Part print with two shaded views. Sizes in mm from the minimum x, y, z corner. A direction names the side the tool comes from. Give positions to 0.01 mm unless a question says otherwise; leave off trailing zeros. Loops run counter-clockwise (first coordinate to the right, second up) from the corner with the lowest first, then second, coordinate; pieces in that order, holes last. Notation, with made-up numbers: (-34, 26.5) -> (-25, 26.5) arc R22 cw to (-25, 38.5) -> close; hole circle Ø2 at (10, 87). An arc over 180 degrees is marked (long way). One line per question, with ' | ' between items.
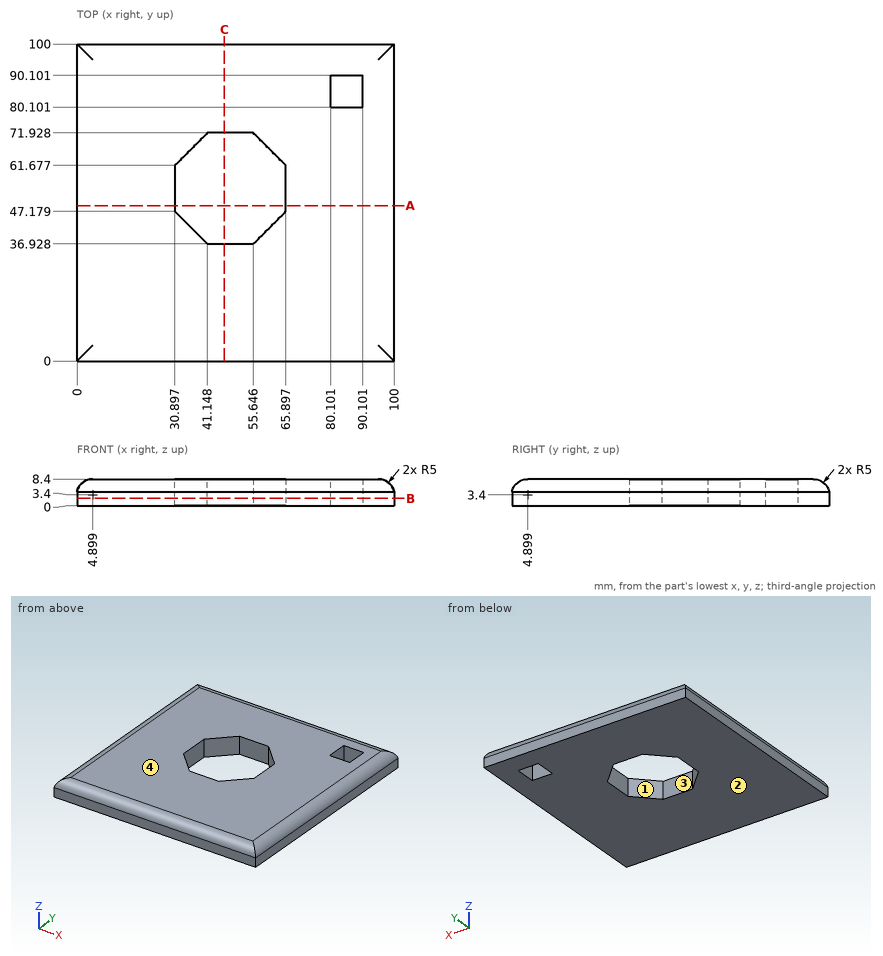
1) Tool access for the marked faces 3 and 4: list every direction of +Z, -Z, +X, -X, +Y, -Y with a clear straight run to the whole face (end or side of a thin tool).
Found:
face 3: +Z, -Z | face 4: +Z, +X, -X, +Y, -Y
2) Pin check, flat tip, straight feed: P1, Ø1, axis at x = 45, z = 5.5, coming from the +Y side. Stop position of the tip, or through.
Found:
P1: y = 99.84
3) Drill centre lines: line 1 (X direction, y = 83.5, z = 3.5); line 2 (Y direction, x = 40, z = 7) (1 decimal). Where is each one in solid material? Low to high.
Found:
line 1: 0 to 80.1, 90.1 to 100 | line 2: 1.4 to 38.1, 70.8 to 98.6
4) Saw through at A-A (y = 49). Give the cut face in (x, z).
Found:
outline: (0, 0) -> (30.9, 0) -> (30.9, 8.4) -> (4.9, 8.4) arc R5 ccw to (0, 4.4) -> close; (65.9, 0) -> (100, 0) -> (100, 4.4) arc R5 ccw to (95.1, 8.4) -> (65.9, 8.4) -> close
5) Pull direction Y, two halves, no side cores. Call the marked faces 1 and 2: pulls with the +Y half, pulls with the -Y half, needs draft (parallel to the pull), parting line crosses it, or undercut.
Found:
face 1: undercut | face 2: needs draft
6) Saw through at B-B (z = 2.25). Give the cut face in (x, y) (1 decimal).
Found:
outline: (0, 0) -> (100, 0) -> (100, 100) -> (0, 100) -> close; hole (30.9, 47.2) -> (41.1, 36.9) -> (55.6, 36.9) -> (65.9, 47.2) -> (65.9, 61.7) -> (55.6, 71.9) -> (41.1, 71.9) -> (30.9, 61.7) -> close; hole (80.1, 80.1) -> (90.1, 80.1) -> (90.1, 90.1) -> (80.1, 90.1) -> close
7) Saw through at C-C (x = 46.5). Give the cut face in (y, z).
Found:
outline: (0, 0) -> (36.93, 0) -> (36.93, 8.4) -> (4.9, 8.4) arc R5 ccw to (0, 4.4) -> close; (71.93, 0) -> (100, 0) -> (100, 4.4) arc R5 ccw to (95.1, 8.4) -> (71.93, 8.4) -> close
